Autodesk Inventor part; units mm, degrees
ref_plane "Arbeitsebene3" through (-12.5, 14, 20) normal (0, 1, 0) x (1, 0, 0)
ref_plane "YZ Plane" through (0, 0, 0) normal (1, 0, 0) x (0, 1, 0)
ref_plane "XZ Plane" through (0, 0, 0) normal (0, 1, 0) x (-1, 0, 0)
sketch "Skizze1" plane through (0, 0, 0) normal (1, 0, 0) x (0, 1, 0)
  line L0 (0, 0) -> (20, 0)
  line L1 (20, 0) -> (20, 20)
  line L2 (20, 20) -> (0, 10.9276)
  line L3 (0, 10.9276) -> (0, 0)
  dimension "d0" = 20
  dimension "d2" = 24.4
  dimension "d18" = 20
extrude "Extrusion1" add sketch "Skizze1" along normal mid plane 25
sketch "Skizze2" plane through (-12.5, 0, 10.9276) normal (0, -0.4131, 0.9107) x (1, 0, 0)
  line L0 (0, 0) -> (0, 21.9615)
  line L1 (0, 21.9615) -> (25, 21.9615)
  line L2 (25, 21.9615) -> (25, 0)
  line L3 (25, 0) -> (0, 0)
  line L4 (0, 21.9615) -> (25, 21.9615)
  line L5 (12.5, 21.9615) -> (12.5, 0) construction
  line L6 (0, 0) -> (25, 0)
  circle A0 centre (5, 8.5) radius 2.35
  circle A1 centre (20, 8.5) radius 2.35
  point P0 (12.5, -4.5142)
  dimension "d5" = 4.7
  dimension "d6" = 15
  dimension "d7" = 8.5
extrude "Extrusion2" cut sketch "Skizze2" against normal blind 5 contours A0 | A1
ref_plane "Arbeitsebene3" through (-12.5, 14, 20) normal (0, 1, 0) x (1, 0, 0)
sketch "Skizze5" plane through (-12.5, 14, 20) normal (0, 1, 0) x (1, 0, 0)
  line L0 (0, 0) -> (25, 0)
  line L1 (25, 20) -> (25, 0)
  line L2 (25, 20) -> (0, 20)
  line L3 (0, 0) -> (0, 20)
  line L4 (12.5, 0) -> (12.5, 20) construction
  line L5 (0, 10) -> (25, 10) construction
  circle A0 centre (12.5, 10) radius 2.7
  circle A1 centre (12.5, 10) radius 4.5
  dimension "d20" = 5.4
  dimension "d21" = 9
extrude "Extrusion5" cut sketch "Skizze5" along normal through all contours A0
extrude "Extrusion6" cut sketch "Skizze5" against normal through all contours A0 | A1
fillet "Rundung1" radius 2 4 edges at (12.5, 0, 5.4638) (12.5, 20, 10) (-12.5, 0, 5.4638) (-12.5, 20, 10)
properties part number "Camera-Mount" material "ABS-Kunststoff"
Can you work these out from the model? Positions are in its coordinate system, mm. A direction names the side the tool comes from. Give positions to 0.01 mm unless a question says otherwise; leave off trailing zeros. Order: outer loops, then holes, each group sorted by start corner. A loop starts at its lowest first (then second) coordinate and runs counter-clockwise, first axis right, second up. Notation, with made-up numbers: (-39, -18) - (-10, -18) arc R14 ccw to (-10, 1) - close; hole circle Ø4 at (-32, 65.25). An arc over 180 degrees is marked (long way). Use a Markdown table: item, result. Add a question column.
Q1. If we section it at A-A on x = 0: Write out the boundary of the cut face in (y, z), plus the area to 3 significant figures.
Q2. If we section it at C-C on y = 17: Write out the boundary of the cut face in (x, z), plus the area to 3 significant figures.
Q3. If we mould it in two halves opening along X, with no side actions, what happens to faces 1 (the flat face through (-2.5, 20, 12.1)), 2 (the cylindrical face through (-0.59, 7.1, 5.54)), 3 (the cylindrical face through (-11.9, 19.43, 10.14))? For each: released by +X, released by -X, zero draft, split by the parting line, or undercut.
Q4. I'm going to push flat-ended pins straight in: pin 1 (10 mm diameter, centred on x = -1.5, z = 11, fed in from -Y); pin 2 (3 mm diameter, centred on x = -0.5, z = 18, fed in from -Y); pin 3 (5 mm diameter, centred on x = 0, z = 10, fed in from +Y). Where does each tip first touch, or does it pass through?
Q5. On a 3-axis mill with a long thin cutter (end or side, diameter ignored), from which of +Z, -Z, +X, -X, +Y, -Y can I reach the whole of each face in a straight line? I mean faces 4 (the flat face through (0, 14, 13)), 5 (the cylindrical face through (-11.9, 0.57, 5.83)), 6 (the flat face through (7.47, 9.84, 9.9)). Say none if no direction works.
Q6. If we section it at B-B on z = 12.25: Count the separate pieces of the cut face and the enclosed holes in it, plus the area to 3 significant figures.
Q7. Please list where these lines run through material, in increasing order: line 1 along X through (y, z) = (4.25, 10); line 2 along X through (y, z) = (16.05, 10); line 3 along X through (y, z) = (7.75, 11.5).
Q8. If we section it at D-D on x = -5.5: Write out the boundary of the cut face in (y, z).
Answers follow:
| question | item | result |
|---|---|---|
| 1 | outline | (0, 0) - (20, 0) - (20, 7.3) - (14, 7.3) - (14, 5.5) - (0, 5.5) - close; (7.88, 14.5) - (14, 14.5) - (14, 12.7) - (20, 12.7) - (20, 20) - close |
| 1 | area | 165 mm^2 |
| 2 | outline | (-12.5, 0) - (12.5, 0) - (12.5, 18.64) - (-12.5, 18.64) - close; hole circle Ø5.4 at (0, 10) |
| 2 | area | 443 mm^2 |
| 3 | face 1 | zero draft |
| 3 | face 2 | undercut |
| 3 | face 3 | released by -X |
| 4 | pin 1 | stops at y = 0 |
| 4 | pin 2 | stops at y = 12.28 |
| 4 | pin 3 | passes through |
| 5 | face 4 | -Y |
| 5 | face 5 | +Z, -Z, -X, -Y |
| 5 | face 6 | none |
| 6 | separate pieces | 2 |
| 6 | enclosed holes | 2 |
| 6 | area | 283 mm^2 |
| 7 | line 1 | x = -12.5 to -4.5, 4.5 to 12.5 |
| 7 | line 2 | x = -12.5 to -2.7, 2.7 to 12.5 |
| 7 | line 3 | x = -12.5 to -9.52, -5.48 to -4.24, 4.24 to 5.48, 9.52 to 12.5 |
| 8 | outline | (0, 0) - (20, 0) - (20, 20) - (8.86, 14.95) - (10.93, 10.39) - (8.68, 9.37) - (6.62, 13.93) - (0, 10.93) - close |
